from build123d import *

# Parameters (mm, degrees)
EXTRUDE_1_DEPTH = 5
CHAMFER_1_SIZE  = 0.8


with BuildPart() as part:
    # Эскиз1 → Повернуть1 (revolve)
    with BuildSketch(Plane.XY, mode=Mode.PRIVATE) as revolve_1_sk:
        with BuildLine():
            Line((-0.723805295, 9), (0, 9))
            Line((0, 9), (0, 4))
            Line((0, 4), (25, 4))
            Line((25, 4), (25, 0))
            Line((25, 0), (-4, 0))
            ThreePointArc((-4, 0), (-3.155479355, 4.78887909), (-0.723805295, 9))
        make_face()
    revolve(revolve_1_sk.sketch.rotate(Axis((-168.009043504, 0, 0), (1, 0, 0)), 90), axis=Axis((-168.009043504, 0, 0), (1, 0, 0)))

    # Эскиз2 → Бобышка-Вытянуть1 (add)
    with BuildSketch(Plane(origin=(0, 0, 0), x_dir=(0, 0, -1), z_dir=(1, 0, 0))):
        Polygon((0, 5.656854249), (-5.656854249, 0), (0, -5.656854249), (5.656854249, 0), align=None)
    extrude(amount=EXTRUDE_1_DEPTH)

    # Эскиз3 → Вырез-Повернуть1 (revolve, cut)
    with BuildSketch(Plane.XY):
        Polygon((5, 4), (4.043414753, 5.656854249), (5, 5.656854249), align=None)
    revolve(axis=Axis((-1000, 0, 0), (1, 0, 0)), mode=Mode.SUBTRACT)

    # Фаска1
    chamfer_1_edges = [part.edges().sort_by_distance(p)[0] for p in [
        (25, 0, -4),
    ]]
    chamfer(chamfer_1_edges, length=CHAMFER_1_SIZE)


solid = part.part
CAD build for the part. Positions are in the model's coordinates, mm. A direction names the side the tool comes from. Give positions to 0.01 mm unless a question says otherwise; leave off trailing zeros. Write each loop counter-clockwise with the first axis right and the second up, starting at its lowest first coordinate (ties: lowest second). Pieces come first, ordered by that corner, then holes. Notation, with made-up numbers: (-32.75, 16.5) - (21.25, 16.5) arc R29 ccw to (21.25, 42.5) - close; hole circle Ø6 at (60.25, 75). An arc over 180 degrees is marked (long way). Put each result on its own line as item: value.
(1) Drop flat-ended pins along their axis: pin 1 Ø1.5 at (x, y) = (-1, -5) entering from -Z; pin 2 Ø2 at (y, z) = (-1, -3.5) entering from -X; pin 3 Ø2 at (y, z) = (-6, 2) entering from -X. Give the stop position or say it passes through.
Working result:
pin 1: z = -7.9
pin 2: x = -3.75
pin 3: x = -2.95
(2) Wall check: L1, parallel to Y at x = -0.5, z = 7; L2, parallel to Z at x = 14.5, y = 0.5; L3, parallel to Y at x = 1, z = 2. Give the ranges that are in metal, low to high.
Working result:
L1: -5.66 to 5.66
L2: -3.97 to 3.97
L3: -3.66 to 3.66
(3) Saw through at C-C (y = -7.5). List the corners of the cut face in (x, z), then the cut area to 3 significant figures.
Working result:
outline: (-0.72, -4.97) - (0, -4.97) - (0, 4.97) - (-0.72, 4.97) arc R11.82 ccw to start
area: 14.6 mm^2
(4) Saw through at B-B (z = -7). List the corners of the cut face in (x, y).
Working result:
outline: (-0.72, -5.66) - (0, -5.66) - (0, 5.66) - (-0.72, 5.66) arc R12.12 ccw to start
(5) Saw through at A-A (x = 22). List the corners of the cut face in (y, z).
Working result:
outline: circle Ø8 at (0, 0)
(6) Tool access for faces 1 (the cylindrical face through (14.734, 3.905, -0.867)), 2 (the flat face through (2.465, 2.868, 2.789)), 3 (the flat face through (2.465, -2.868, -2.789)), 4 (the flat face through (2.465, -2.789, 2.868)): list every direction of +Z, -Z, +X, -X, +Y, -Y with a clear straight run to the whole face (end or side of a thin tool).
Working result:
face 1: +X
face 2: +Z, +X, +Y
face 3: -Z, +X, -Y
face 4: +Z, +X, -Y
